Verification items for the finished model (mm, model axes). Round coordinates to 2 decimals unless told otherwise and drop trailing zeros. Write each loop counter-clockwise with the first axis right and the second up, starting at its lowest first coordinate (ties: lowest second). Pieces come first, ordered by that corner, then holes. Notation, with made-up numbers: (85, -30.75) - (110, -30.75) arc R21 cw to (110, 4.25) - close; hole circle Ø11 at (22.5, 87). An arc over 180 degrees is marked (long way). Answer as a JSON object with one key per item and string values.
```python
from build123d import *

# Parameters (mm, degrees)
SALIENTE_EXTRUIR1_DEPTH = 3
CROQUIS2_R              = 1.55
CORTAR_EXTRUIR1_DEPTH   = 3
CROQUIS4_W              = 3
CROQUIS4_H              = 12.805
CORTAR_EXTRUIR2_DEPTH   = 10


with BuildPart() as part:
    # Model → Saliente-Extruir1 (new body)
    with BuildSketch(Plane.XY):
        Polygon((186, 103), (186, 90.195), (183, 90.195), (183, 65.805), (186, 65.805), (186, 53), (220.805, 53), (220.805, 56), (245.195, 56), (245.195, 53), (269.585, 53), (280, 53), (280, 65.805), (283, 65.805), (283, 90.195), (280, 90.195), (280, 103), align=None)
    extrude(amount=SALIENTE_EXTRUIR1_DEPTH)

    # Croquis2 → Cortar-Extruir1 (cut)
    with BuildSketch(Plane.XY.offset(3)):
        with Locations((233, 78)):
            Circle(CROQUIS2_R)
        with Locations((198, 78)):
            Circle(CROQUIS2_R)
    extrude(amount=-CORTAR_EXTRUIR1_DEPTH, mode=Mode.SUBTRACT)

    # Croquis4 → Cortar-Extruir2 (cut)
    with BuildSketch(Plane.XY.offset(3)):
        with Locations((278.5, 96.5975)):
            Rectangle(CROQUIS4_W, CROQUIS4_H)
        with Locations((278.5, 59.4025)):
            Rectangle(CROQUIS4_W, CROQUIS4_H)
    extrude(amount=-CORTAR_EXTRUIR2_DEPTH, mode=Mode.SUBTRACT)


solid = part.part
```
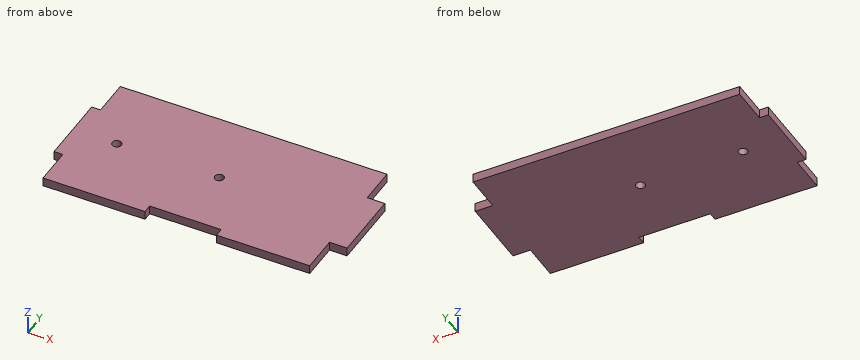
1. Cross-section at B-B (z = 2.25). Record the boundary of the cut face in (x, y) (3 decimals).
Completed:
{"outline": "(183, 65.805) - (186, 65.805) - (186, 53) - (220.805, 53) - (220.805, 56) - (245.195, 56) - (245.195, 53) - (277, 53) - (277, 65.805) - (283, 65.805) - (283, 90.195) - (277, 90.195) - (277, 103) - (186, 103) - (186, 90.195) - (183, 90.195) - close; hole circle Ø3.1 at (198, 78); hole circle Ø3.1 at (233, 78)"}
2. Cross-section at A-A (x = 198). Record the boundary of the cut face in (y, z), plus the area to 3 significant figures.
Completed:
{"outline": "(53, 0) - (76.45, 0) - (76.45, 3) - (53, 3) - close; (79.55, 0) - (103, 0) - (103, 3) - (79.55, 3) - close", "area": "141 mm^2"}
3. Cross-section at C-C (y = 78). Record the boundary of the cut face in (x, z).
Completed:
{"outline": "(183, 0) - (196.45, 0) - (196.45, 3) - (183, 3) - close; (199.55, 0) - (231.45, 0) - (231.45, 3) - (199.55, 3) - close; (234.55, 0) - (283, 0) - (283, 3) - (234.55, 3) - close"}
4. Cross-section at D-D (x = 233). Record the boundary of the cut face in (y, z), plus the area to 3 significant figures.
Completed:
{"outline": "(56, 0) - (76.45, 0) - (76.45, 3) - (56, 3) - close; (79.55, 0) - (103, 0) - (103, 3) - (79.55, 3) - close", "area": "132 mm^2"}
5. Material ranges on probe 1 along X at (y, z) = (78, 1.9); probe 2 along Y at (x, z) = (233, 2); probe 3 along Y at (x, z) = (230, 1.3), recorded low to high. Write a range as from..to.
Completed:
{"probe 1": "x = 183..196.45, 199.55..231.45, 234.55..283", "probe 2": "y = 56..76.45, 79.55..103", "probe 3": "y = 56..103"}
6. Go/stop test with flat-tipped pins: pin 1 (1.5 mm diameter, centred on x = 185, z = 2, fed in from -Y) (3 decimals); pin 2 (1.5 mm diameter, centred on y = 57.5, z = 1, fed in from -X); pin 3 (0.9 mm diameter, centred on x = 279, z = 1, fed in from +Y) (3 decimals). Record where each tip stops, or that it passes through.
Completed:
{"pin 1": "stops at y = 65.805", "pin 2": "stops at x = 186", "pin 3": "stops at y = 90.195"}
